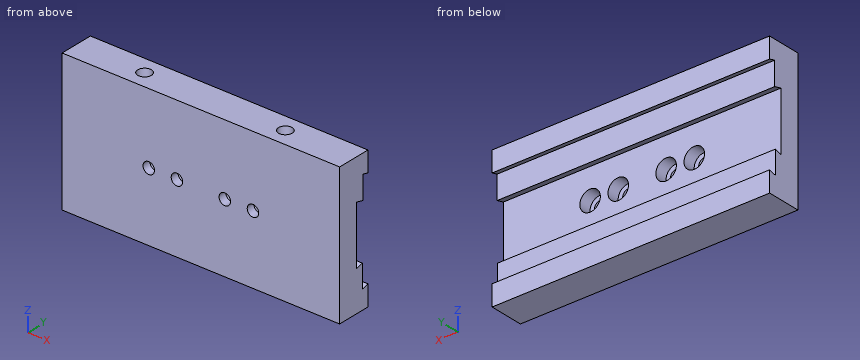
Autodesk Inventor part; units mm, degrees
ref_plane "YZ Plane" through (0, 0, 0) normal (1, 0, 0) x (0, 1, 0)
ref_plane "XZ Plane" through (0, 0, 0) normal (0, 1, 0) x (-1, 0, 0)
ref_plane "XY Plane" through (0, 0, 0) normal (0, 0, 1) x (1, 0, 0)
sketch "Sketch1" plane through (0, 0, 0) normal (1, 0, 0) x (0, 1, 0)
  line L0 (-13.4609, 51.6064) -> (11.5391, 51.6064)
  line L1 (11.5391, -50.3936) -> (-13.4609, -50.3936)
  line L2 (-13.4609, -50.3936) -> (-13.4609, 51.6064)
  line L3 (-13.4609, 51.6064) -> (11.5391, -50.3936) construction
  line L4 (11.5391, 51.6064) -> (-13.4609, -50.3936) construction
  line L5 (1.5391, 22.1864) -> (1.5391, -20.9936)
  line L6 (7.1158, 37.8541) -> (11.5391, 36.6689)
  line L7 (6.5391, -36.6436) -> (11.5391, -35.3039)
  line L8 (6.5391, -36.6436) -> (13.9505, -36.6436) construction
  line L9 (1.5391, 22.1864) -> (7.1158, 20.6921)
  line L10 (1.5391, -20.9936) -> (6.5391, -19.6539)
  line L11 (7.1158, 37.8541) -> (7.1158, 20.6921)
  line L12 (6.5391, -19.6539) -> (6.5391, -36.6436)
  line L13 (11.5391, 51.6064) -> (11.5391, 36.6689)
  line L14 (11.5391, -35.3039) -> (11.5391, -50.3936)
  point P0 (-0.9609, 0.6064)
  dimension "d2" = 25
  dimension "d3" = 102
  dimension "d4" = 43.18
  dimension "d5" = 21.6
  dimension "d6" = 74.5
  dimension "d7" = 37.25
  dimension "d10" = 15
  dimension "d43" = 75
extrude "Extrusion1" add sketch "Sketch1" along normal blind 203
sketch "Sketch2" plane through (0, 1.5391, 22.1864) normal (0, 1, 0) x (1, 0, 0)
  point P0 (0, 22.1864)
  point P1 (63.4, 22.1864)
  point P2 (139.6, 22.1864)
  dimension "d14" = 76.2
  dimension "d15" = 63.4
hole "Hole1" at (63.4, 1.5391, 0) at (139.6, 1.5391, 0) direction (0, -1, 0) diameter 8.4 end through all counterbore diameter 15 counterbore depth 9
sketch "Sketch3" plane through (0, 1.5391, 22.1864) normal (0, 1, 0) x (1, 0, 0)
  point P0 (0, 22.1864)
  point P1 (84, 22.1864)
  point P2 (119, 22.1864)
  dimension "d23" = 35
  dimension "d24" = 84
hole "Hole2" at (84, 1.5391, 0) at (119, 1.5391, 0) direction (0, -1, 0) diameter 8.4 end through all counterbore diameter 15 counterbore depth 9
sketch "Sketch4" plane through (0, -13.4609, 51.6064) normal (0, 0, 1) x (1, 0, 0)
  line L0 (0, 0) -> (203, 0)
  line L1 (0, 0) -> (0, 25)
  line L2 (203, 25) -> (203, 0)
  point P0 (0, 13.4609)
  point P1 (50, 12.5)
  point P2 (153, 12.5)
  dimension "d32" = 12.5
  dimension "d33" = 12.5
  dimension "d34" = 50
  dimension "d35" = 50
hole "Hole3" at (50, -0.9609, 51.6064) at (153, -0.9609, 51.6064) direction (0, 0, -1) diameter 10 depth 10 tip angle 118
properties part number "czescuchwytu" material "Iron, Cast"
Read the model definition and answer for the solid it produces. Units are mm, in the model's axes. Coordinates: 2 decimals unless noted, no trailing zeros. Loops run counter-clockwise (first coordinate to the right, second up) from the corner with the lowest first, then second, coordinate; pieces in that order, holes last.
(1) The part is cut by section D-D (z = -15). Determine the outline of the cut face in (x, y).
Solution:
outline: (0, -13.46) - (203, -13.46) - (203, 1.54) - (0, 1.54) - close
(2) Flat-ended cylindrical pins translate along their axes: pin 1 Ø9 at (x, z) = (139.6, 0) entering from +Y; pin 2 Ø16.5 at (x, z) = (136.5, -1) entering from +Y; pin 3 Ø1.5 at (x, z) = (171, -34.5) entering from +Y. Find the tip coordinate at first contact, or state that the pin passes through.
Solution:
pin 1: stops at y = -7.46
pin 2: stops at y = 1.54
pin 3: stops at y = 6.54
(3) The part is cut by section A-A (x = 139.6). Determine the outline of the cut face in (y, z).
Solution:
outline: (-13.46, -50.39) - (11.54, -50.39) - (11.54, -35.3) - (6.54, -36.64) - (6.54, -19.65) - (1.54, -20.99) - (1.54, -7.5) - (-7.46, -7.5) - (-7.46, -4.2) - (-13.46, -4.2) - close; (-13.46, 4.2) - (-7.46, 4.2) - (-7.46, 7.5) - (1.54, 7.5) - (1.54, 22.19) - (7.12, 20.69) - (7.12, 37.85) - (11.54, 36.67) - (11.54, 51.61) - (-13.46, 51.61) - close
(4) The part is cut by section C-C (x = 183.5). Determine the outline of the cut face in (y, z).
Solution:
outline: (-13.46, -50.39) - (11.54, -50.39) - (11.54, -35.3) - (6.54, -36.64) - (6.54, -19.65) - (1.54, -20.99) - (1.54, 22.19) - (7.12, 20.69) - (7.12, 37.85) - (11.54, 36.67) - (11.54, 51.61) - (-13.46, 51.61) - close
(5) Consider line 1 along X through (y, z) = (-4.5, 0); line 2 along Z through (x, y) = (63.4, -4.25); line 3 along Z through (x, y) = (63.4, -11.5). Determine where each line is inside the solid, lowest interval first.
Solution:
line 1: x = 0 to 55.9, 70.9 to 76.5, 91.5 to 111.5, 126.5 to 132.1, 147.1 to 203
line 2: z = -50.39 to -7.5, 7.5 to 51.61
line 3: z = -50.39 to -4.2, 4.2 to 51.61
(6) The part is cut by section B-B (z = 0). Count the separate pieces of the cut face and the enclosed holes in it, and give its area (3 significant figures).
Solution:
separate pieces: 5
enclosed holes: 0
area: 2,300 mm2
